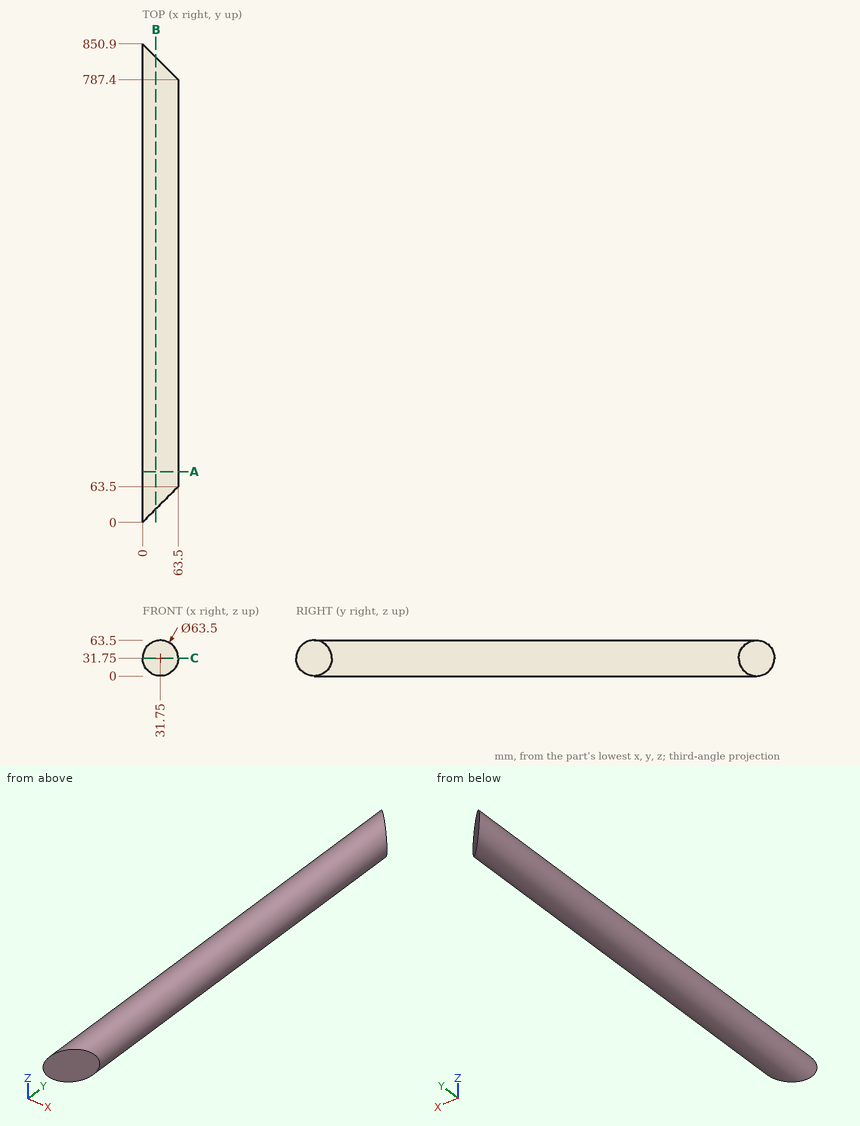
The drawing under review shows one solid part. Ordinate dimensions are in mm from its lowest x, y, z. Round coordinates to 2 decimals unless told otherwise and drop trailing zeros. Loops run counter-clockwise (first coordinate to the right, second up) from the corner with the lowest first, then second, coordinate; pieces in that order, holes last. Notation, with made-up numbers: M 48.25,15.5 L 53.25,15.5 A14 cw 53.25,22.5 Z; hole C -7,0 d9. An arc over 180 degrees is marked long. Answer as CSV lines item,"result". Start each with the question number.
Item 1: Consider section C-C (z = 31.75). Write out the cut boundary in (x, y), then the cut area to 3 significant figures.
Item 2: Consider section A-A (y = 90). Write out the cut boundary in (x, z).
Item 3: Insertion check: P1, Ø10, axis at x = 9, z = 36.5, coming from the +Y side; P2, Ø4, axis at x = 38, y = 631.5, coming from the +Z side; P3, Ø10, axis at x = 48.5, z = 14.5, coming from the -Y side. Each pin has a flat end and moves straight along its axis. Give the tip position at first contact, or say it passes through.
Item 4: Wall thickness on line 1 (X direction, y = 647, z = 30.5); line 2 (Z direction, x = 31, y = 776); line 3 (Z direction, x = 34, y = 378): over which ranges is each line inside the solid? List them lowest first. Write a range as [from, to].
Item 5: Consider section B-B (x = 24). Write out the cut boundary in (y, z), then the cut area to 3 significant figures.
Answer:
1,outline,"M 0,0 L 63.5,63.5 L 63.5,787.4 L 0,850.9 Z"
1,area,"50,000 mm^2"
2,outline,"C 31.75,31.75 d63.5"
3,P1,"stops at y = 846.9"
3,P2,"stops at z = 63.21"
3,P3,"stops at y = 43.5"
4,line 1,"x = [0.02, 63.48]"
4,line 2,"z = [0.01, 63.49]"
4,line 3,"z = [0.08, 63.42]"
5,outline,"M 24,0.96 L 826.9,0.96 L 826.9,62.54 L 24,62.54 Z"
5,area,"49,400 mm^2"
